Input: part model. Units: mm. Frame: model coordinates. A direction names the side the tool comes from. Coordinates: 2 decimals unless noted, no trailing zeros. Loops run counter-clockwise (first coordinate to the right, second up) from the corner with the lowest first, then second, coordinate; pieces in that order, holes last.
Item 1: Pull-direction query (Z, two-part tool) for faces 3 (the cylindrical face through (-3.417, 0.309, -0.759)), 4 (the cylindrical face through (0.03, 3.2, 2.15)), 5 (the flat face through (0, 7.5, 0)); classes: released by +Z, released by -Z, zero draft, split by the parting line, or undercut.
Item 2: Contact query for flat-ended pins moving along their axis: P1, Ø2, axis at x = 4, y = 4.5, coming from the -Z side; P2, Ø2, axis at y = 5, z = -3.5, coming from the +X side; P3, Ø3, axis at x = -3, y = 2, coming from the +Z side. Output: stop coordinate, or through.
Item 3: Section B-B on y = 1. Return loops of the section in (x, z) (3 decimals).
Item 4: Reachability of faces 1 (the flat face through (-1.625, 3, 0)), 2 (the flat face through (-2, 0, -2)) from +Z, -Z, +X, -X, +Y, -Y: full face, straight path, thin tool, end or side. Return the list, or none.
Item 5: Section A-A on y = 6. Return loops of the section in (x, z) (3 decimals), and give its area (3 significant figures).
Item 6: Ray query, line 1 along X through (y, z) = (2, -0.25) (3 decimals); line 2 along Z through (x, y) = (-0.5, 0.5); line 3 along X through (y, z) = (3, 0.25) (3 decimals). Return the intervals inside material, ascending.
```python
from build123d import *

# Parameters (mm, degrees)
SKETCH_1_R          = 3.5
EXTRUDE_1_DEPTH     = 4.5
SKETCH_2_R          = 6.5
EXTRUDE_2_DEPTH     = 3
FILLET_1_R          = 2.5
FILLET_2_R          = 4
SKETCH_3_W          = 3.25
SKETCH_3_H          = 2.815581646
CUT_EXTRUDE_1_DEPTH = 6.5
FILLET_3_R          = 1


with BuildPart() as part:
    # 草图1 → 凸台-拉伸1 (new body)
    with BuildSketch(Plane(origin=(0, 0, 0), x_dir=(1, 0, 0), z_dir=(0, 1, 0))):
        with Locations(Location((0, 0, 0), (0, 0, 270))):
            Circle(SKETCH_1_R)
    extrude(amount=EXTRUDE_1_DEPTH)

    # 草图2 → 凸台-拉伸2 (add)
    with BuildSketch(Plane(origin=(0, 4.5, 0), x_dir=(1, 0, 0), z_dir=(0, 1, 0))):
        with Locations(Location((0, 0, 0), (0, 0, 270))):
            Circle(SKETCH_2_R)
    extrude(amount=EXTRUDE_2_DEPTH)

    # 圆角1
    fillet_1_edges = [part.edges().sort_by_distance(p)[0] for p in [
        (0, 7.5, -6.5),
    ]]
    fillet(fillet_1_edges, radius=FILLET_1_R)

    # 圆角2
    # the kernel refuses this fillet: 4 mm, written as the material it adds along each edge
    with BuildSketch(Plane(origin=(0, 4.5, 0), x_dir=(0, 0, 1), z_dir=(-1, 0, 0))) as fillet_2_piece_1:
        with BuildLine():
            CenterArc((7.5, -3.872983346), FILLET_2_R, 104.477512186, 75.522487814)
            Line((3.5, -3.872983346), (3.42, -3.872983346))
            Line((3.42, -3.872983346), (3.42, 0))
            Line((3.42, 0), (3.5, 0.08))
            ThreePointArc((3.5, 0.08), (5, 0.08), (6.48, 0.077459667))
            Line((6.48, 0.077459667), (6.5, 0))
        make_face()
    revolve(axis=Axis((0, 4.5, 0), (0, 1, 0)))

    # 草图3 → 切除-拉伸1 (cut)
    with BuildSketch(Plane.XZ):
        with BuildLine():
            ThreePointArc((1.625, 1.407790823), (0, 2.15), (-1.625, 1.407790823))
            Line((-1.625, 1.407790823), (1.625, 1.407790823))
        make_face()
        Rectangle(SKETCH_3_W, SKETCH_3_H)
        with BuildLine():
            Line((1.625, -1.407790823), (-1.625, -1.407790823))
            ThreePointArc((-1.625, -1.407790823), (0, -2.15), (1.625, -1.407790823))
        make_face()
    extrude(amount=-CUT_EXTRUDE_1_DEPTH, mode=Mode.SUBTRACT)

    # 圆角3
    fillet_3_edges = [part.edges().sort_by_distance(p)[0] for p in [
        (0, 4.5, -6.5),
    ]]
    fillet(fillet_3_edges, radius=FILLET_3_R)


solid = part.part
```
Results found:
1. face 3: split by the parting line
1. face 4: undercut
1. face 5: zero draft
2. P1: stops at z = -5.66
2. P2: stops at x = 5.98
2. P3: stops at z = 3.92
3. outline: circle Ø7.035 at (0, 0); hole (-1.625, -1.408) arc R2.15 ccw to (1.625, -1.408) - (1.625, 1.408) arc R2.15 ccw to (-1.625, 1.408) - close
4. face 1: -Y
4. face 2: +Z, -Z, +X, -X, -Y
5. outline: circle Ø12.583 at (0, 0); hole (-1.625, -1.408) arc R2.15 ccw to (1.625, -1.408) - (1.625, 1.408) arc R2.15 ccw to (-1.625, 1.408) - close
5. area: 112 mm2
6. line 1: x = -3.735 to -1.625, 1.625 to 3.735
6. line 2: z = -3.46 to -2.09, 2.09 to 3.46
6. line 3: x = -4.273 to -1.625, 1.625 to 4.273
